The model under review builds one solid part; all positions refer to its coordinate system, in mm. Face numbers are marked on the shaded views. Coordinates: 2 decimals unless noted, no trailing zeros. Write each loop counter-clockwise with the first axis right and the second up, starting at its lowest first coordinate (ties: lowest second). Pieces come first, ordered by that corner, then holes. Notation, with made-up numbers: (-16, -31.5) - (15, -31.5) arc R23 cw to (15, 4.5) - close; hole circle Ø4 at (27, 43.25). An arc over 180 degrees is marked (long way). Return JSON: item names as keys, results as strings. Group by question number.
(1) We need section D-D on z = 2.75. State the section outline as (x, y) points, then the cut area to 3 significant figures.
(2) For pin 1 Ø2 at (x, z) = (-2.5, 4.5) entering from +Y; pin 2 Ø1.5 at (x, y) = (-2.5, 3) entering from -Z; pin 3 Ø2 at (x, z) = (4.5, 4) entering from -Y; pin 4 Ø2 at (x, z) = (3.5, 1.5) entering from -Y, all flat-tipped, find the tip position at first contact; note any pin that passes through.
(3) We need section C-C on z = 5.5. State the section outline as (x, y) points, then the cut area to 3 significant figures.
(4) Draft analysis for pull direction Y (two halves, no side actions). For the marked faces 1, 2, 3 and 4, state which applies: released by +Y, released by -Y, zero draft, split by the parting line, or undercut.
(5) To check wall thickness, follow L1, parallel to Y at x = 0, z = 4.15; L2, parallel to Z at x = -2.75, y = 4; L3, parallel to X at y = -1, z = 3.75. State the ranges of each line that lie inside material, in increasing order. Write a range as from..to.
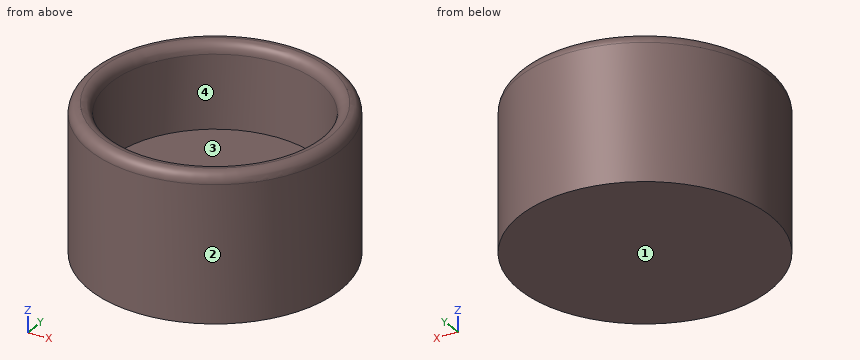
```python
from build123d import *

# Parameters (mm, degrees)
F0_R     = 6
F0_R_2   = 5
F1_DEPTH = 7
F2_DEPTH = 3
F3_R     = 0.49999


# Not quite as in the source:
# - a fillet or chamfer is up to 0.001 mm smaller than in the source, because OpenCascade refuses the exact size


with BuildPart() as f1:
    # F0 (on Top) → F1 (new body)
    with BuildSketch(Plane.XY):
        Circle(F0_R)
        Circle(F0_R_2, mode=Mode.SUBTRACT)
    extrude(amount=F1_DEPTH)

    # F0 (on Top) → F2 (join)
    with BuildSketch(Plane.XY):
        Circle(F0_R_2)
    extrude(amount=F2_DEPTH)

    # F3 (radius 0.5 in the source; OpenCascade refuses exactly that, so slightly less here)
    f3_edges = [f1.edges().sort_by_distance(p)[0] for p in [
        (-6, 0, 7),
        (-5, 0, 7),
    ]]
    fillet(f3_edges, radius=F3_R)


solid = f1.part
```
Ans:
{
 "1": {"outline": "circle Ø12 at (0, 0)", "area": "113 mm²"},
 "2": {"pin 1": "y = 5.81", "pin 2": "z = 0", "pin 3": "y = -4.87", "pin 4": "y = -5.45"},
 "3": {"outline": "circle Ø12 at (0, 0); hole circle Ø10 at (0, 0)", "area": "34.6 mm²"},
 "4": {"face 1": "zero draft", "face 2": "split by the parting line", "face 3": "undercut", "face 4": "undercut"},
 "5": {"L1": "-6..-5, 5..6", "L2": "0..3", "L3": "-5.92..-4.9, 4.9..5.92"}
}
